For this review, use the dimensioned drawing (mm, ordinates from the lowest corner) and the shaded views. A direction names the side the tool comes from. Round coordinates to 2 decimals unless told otherwise and drop trailing zeros. Loops run counter-clockwise (first coordinate to the right, second up) from the corner with the lowest first, then second, coordinate; pieces in that order, holes last. Notation, with made-up numbers: M -3.5,47.25 L 11.5,47.25 A21 cw 11.5,70.25 Z; hole C -25.75,54.25 d11. An arc over 180 degrees is marked long. One line per item, written item: value. Start each with the question number.
Item 1: Clearance check with flat-ended pins moving along their axes: pin 1 (14 mm diameter, centred on x = 22.5, z = 19.5, fed in from +Y); pin 2 (10 mm diameter, centred on x = 15, z = 28, fed in from +Y); pin 3 (12 mm diameter, centred on x = 7, z = 6, fed in from +Y); pin 4 (12 mm diameter, centred on y = 19.5, z = 22, fed in from -X). State where each tip first meets the part, or that it passes through.
Item 2: For line 1 along Y through (x, z) = (23, 4.5); line 2 along Z through (x, y) = (38, 62.5); line 3 along Z through (x, y) = (42, 12) (1 decimal), list the stretches that pass through material, from the lowest coordinate up.
Item 3: We need section C-C (y = 63.5). Write out the cut boundary in (x, z).
Item 4: We need section D-D (y = 49.5). Write out the cut boundary in (x, z), then the cut area to 3 significant figures.
Item 5: We need section B-B (x = 17.5). Write out the cut boundary in (y, z), then the cut area to 3 significant figures.
Item 6: We need section A-A (z = 16.5). Write out the cut boundary in (x, y) (1 decimal), then the cut area to 3 significant figures.
Item 7: For the marked faces 1 and 2, list the 3-axis set-ups (+Z, -Z, +X, -X, +Y, -Y) from which the entire face can be reached by the end or side of a thin tool; tool diameter is ignored.
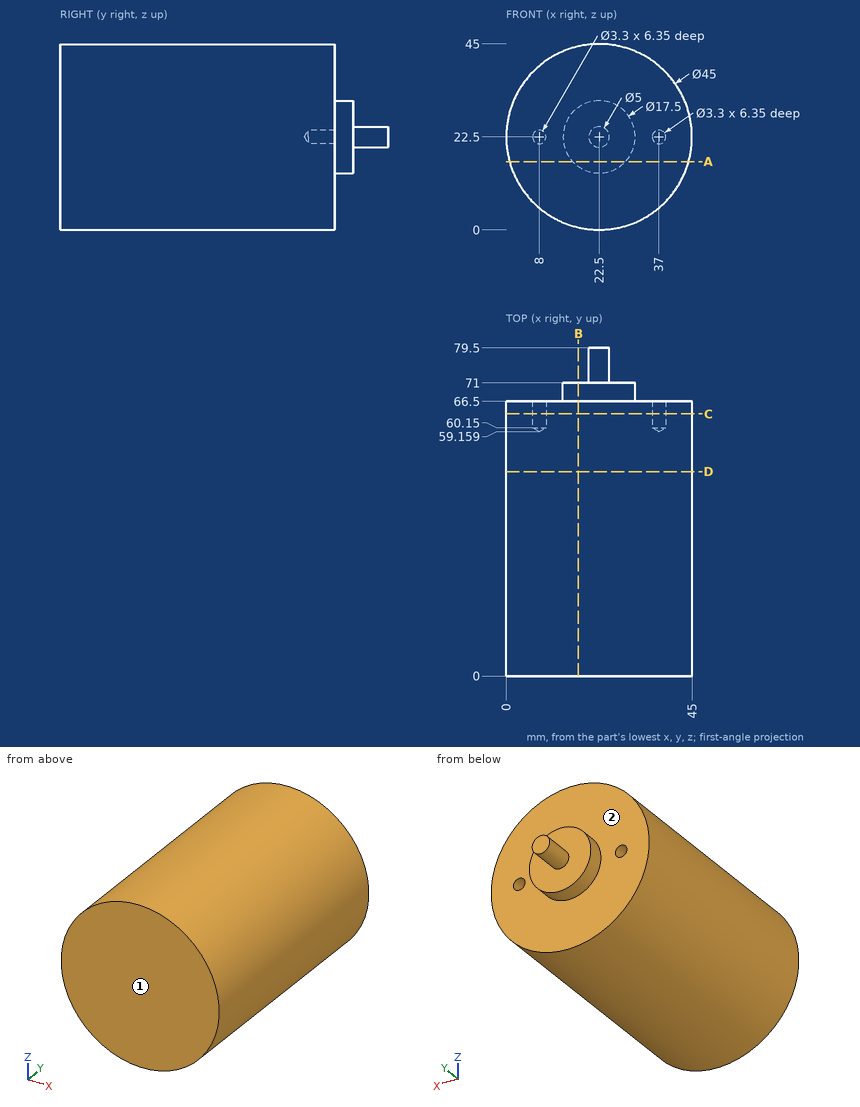
A:
1. pin 1: y = 79.5
1. pin 2: y = 71
1. pin 3: y = 66.5
1. pin 4: x = 0
2. line 1: 0 to 66.5
2. line 2: 6.19 to 21.19, 23.81 to 38.81
2. line 3: 11.3 to 33.7
3. outline: C 22.5,22.5 d45; hole C 8,22.5 d3.3; hole C 37,22.5 d3.3
4. outline: C 22.5,22.5 d45
4. area: 1,590 mm2
5. outline: M 0,0.56 L 66.5,0.56 L 66.5,15.32 L 71,15.32 L 71,29.68 L 66.5,29.68 L 66.5,44.44 L 0,44.44 Z
5. area: 2,980 mm2
6. outline: M 0.8,0 L 44.2,0 L 44.2,66.5 L 28.9,66.5 L 28.9,71 L 16.1,71 L 16.1,66.5 L 0.8,66.5 Z
6. area: 2,940 mm2
7. face 1: +Z, -Z, +X, -X, -Y
7. face 2: +Y
